The model under review builds one solid part; all positions refer to its coordinate system, in mm. A direction names the side the tool comes from. Round coordinates to 2 decimals unless told otherwise and drop trailing zeros. Write each loop counter-clockwise with the first axis right and the second up, starting at its lowest first coordinate (ties: lowest second). Pieces come first, ordered by that corner, then holes.
Item 1: Add section A-A (y = 9.5). Give the boundary of the cut face in (x, z).
Item 2: Machinability: for faces 5 (the face through (-96, -3.863, 2)), 6 (the face through (-38, 34, 0)), 7 (the face through (-36, -30.276, 2)), which of the approach directions +Z, -Z, +X, -X, +Y, -Y give a long, thin tool a straight path to every point of the face, cutting with its end or side? Answer none if there is none.
Item 3: To check wall thickness, follow L1, parallel to Y at x = -64, z = 3.15; L2, parallel to X at y = 54, z = 1.35; L3, parallel to X at y = 34.5, z = 3.25. State the ranges of each line that lie inside material, in increasing order.
Item 4: Add section D-D (x = -30). Give the boundary of the cut face in (y, z).
Item 5: Add section B-B (x = -85). Give the boundary of the cut face in (y, z), plus the area to 3 significant figures.
Item 6: Add section C-C (z = 2.4). Give the boundary of the cut face in (x, y), plus the area to 4 significant figures.
Item 7: Draft analysis for pull direction X (two halves, no side actions). For faces 1 (the face through (100, -1, 2)), 2 (the face through (-38, 34, 4)), 3 (the face through (-63, -33.276, 2)), 4 (the face through (-100, -40, 2)), state which applies: +X half, -X half, draft (parallel to the pull), parting line (faces both ways), or undercut.
```python
from build123d import *

# Parameters (mm, degrees)
F0_W     = 200
F0_H     = 150
F1_DEPTH = 4
F2_W     = 10
F2_H     = 12.5
F3_DEPTH = 25


with BuildPart() as f1:
    # F0 (on Top) → F1 (new body)
    with BuildSketch(Plane.XY):
        Rectangle(F0_W, F0_H)
    extrude(amount=F1_DEPTH)

    # F2 (on face) → F3 (cut)
    with BuildSketch(Plane.XY.offset(4)):
        Polygon((87.4994372893, -64.5627596692), (87.4994372893, 60.4372403308), (-87.5005627107, 60.4372403308), (-87.5005627107, 34.7239444211), (-41.0005627107, 34.7239444211), (-33.5005627107, 34.7239444211), (-33.5005627107, 26.7239444211), (-38.5005627107, 26.7239444211), (-38.5005627107, 29.7239444211), (-46.0005627107, 29.7239444211), (-87.5005627107, 29.7239444211), (-87.5005627107, 2.7372403308), (-92.5005627107, -0.2627596692), (-100, -0.2627596692), (-100, -3.8627596692), (-92.5005627107, -3.8627596692), (-87.5005627107, -6.8627596692), (-87.5005627107, -33.2760555789), (-38.5005627107, -33.2760555789), (-38.5005627107, -30.2760555789), (-33.5005627107, -30.2760555789), (-33.5005627107, -38.2760555789), (-41.0005627107, -38.2760555789), (-46.0005627107, -38.2760555789), (-87.5005627107, -38.2760555789), (-87.5005627107, -64.5627596692), (-77.5005627107, -64.5627596692), align=None)
        with BuildLine():
            Line((-77.3623862099, 50.4372403308), (-74.3623862099, 50.4372403308))
            Line((-74.3623862099, 50.4372403308), (60.6376137901, 50.4372403308))
            Line((60.6376137901, 50.4372403308), (74.4994372893, 50.4372403308))
            Line((74.4994372893, 50.4372403308), (77.4994372893, 50.4372403308))
            Line((77.4994372893, 50.4372403308), (77.4994372893, 47.4372403308))
            Line((77.4994372893, 47.4372403308), (77.4994372893, -54.5627596692))
            Line((77.4994372893, -54.5627596692), (60.6376137901, -54.5627596692))
            Line((60.6376137901, -54.5627596692), (-77.5005627107, -54.5627596692))
            Line((-77.5005627107, -54.5627596692), (-77.5005627107, -51.5627596692))
            Line((-77.5005627107, -51.5627596692), (60.6376137901, -51.5627596692))
            Line((60.6376137901, -51.5627596692), (69.4994372893, -51.5627596692))
            ThreePointArc((69.4994372893, -51.5627596692), (73.0349711952, -50.0982935751), (74.4994372893, -46.5627596692))
            Line((74.4994372893, -46.5627596692), (74.4994372893, 42.4372403308))
            ThreePointArc((74.4994372893, 42.4372403308), (73.0349711952, 45.9727742368), (69.4994372893, 47.4372403308))
            Line((69.4994372893, 47.4372403308), (60.6376137901, 47.4372403308))
            Line((60.6376137901, 47.4372403308), (57.6376137901, 47.4372403308))
            Line((57.6376137901, 47.4372403308), (-74.3623862099, 47.4372403308))
            Line((-74.3623862099, 47.4372403308), (-77.3623862099, 47.4372403308))
            Line((-77.3623862099, 47.4372403308), (-77.3623862099, 50.4372403308))
        make_face(mode=Mode.SUBTRACT)
        Polygon((39.9994372893, -27.0627596692), (39.9994372893, -2.0627596692), (39.9994372893, 22.9372403308), (39.9994372893, 35.4372403308), (49.9994372893, 35.4372403308), (49.9994372893, 22.9372403308), (49.9994372893, -27.0627596692), (49.9994372893, -39.5627596692), (39.9994372893, -39.5627596692), align=None, mode=Mode.SUBTRACT)
        with BuildLine():
            Line((60.6376137901, 50.4372403308), (-74.3623862099, 50.4372403308))
            Line((-74.3623862099, 50.4372403308), (-77.3623862099, 50.4372403308))
            Line((-77.3623862099, 50.4372403308), (-77.3623862099, 47.4372403308))
            Line((-77.3623862099, 47.4372403308), (-74.3623862099, 47.4372403308))
            Line((-74.3623862099, 47.4372403308), (57.6376137901, 47.4372403308))
            Line((57.6376137901, 47.4372403308), (60.6376137901, 47.4372403308))
            Line((60.6376137901, 47.4372403308), (69.4994372893, 47.4372403308))
            ThreePointArc((69.4994372893, 47.4372403308), (73.0349711952, 45.9727742368), (74.4994372893, 42.4372403308))
            Line((74.4994372893, 42.4372403308), (74.4994372893, -46.5627596692))
            ThreePointArc((74.4994372893, -46.5627596692), (73.0349711952, -50.0982935751), (69.4994372893, -51.5627596692))
            Line((69.4994372893, -51.5627596692), (60.6376137901, -51.5627596692))
            Line((60.6376137901, -51.5627596692), (-77.5005627107, -51.5627596692))
            Line((-77.5005627107, -51.5627596692), (-77.5005627107, -54.5627596692))
            Line((-77.5005627107, -54.5627596692), (60.6376137901, -54.5627596692))
            Line((60.6376137901, -54.5627596692), (77.4994372893, -54.5627596692))
            Line((77.4994372893, -54.5627596692), (77.4994372893, 47.4372403308))
            Line((77.4994372893, 47.4372403308), (77.4994372893, 50.4372403308))
            Line((77.4994372893, 50.4372403308), (74.4994372893, 50.4372403308))
            Line((74.4994372893, 50.4372403308), (60.6376137901, 50.4372403308))
        make_face()
        with Locations((44.9994372893, 29.1872403308)):
            Rectangle(F2_W, F2_H)
        Polygon((39.9994372893, 22.9372403308), (39.9994372893, -2.0627596692), (39.9994372893, -27.0627596692), (49.9994372893, -27.0627596692), (49.9994372893, 22.9372403308), align=None)
        with Locations((44.9994372893, -33.3127596692)):
            Rectangle(F2_W, F2_H)
    extrude(amount=-F3_DEPTH, mode=Mode.SUBTRACT)


solid = f1.part
```
Numbers:
1. outline: (-100, 0) - (-87.5, 0) - (-87.5, 4) - (-100, 4) - close; (87.5, 0) - (100, 0) - (100, 4) - (87.5, 4) - close
2. face 5: +Z, -Z, -X
2. face 6: -Z, +X, -X, +Y, -Y
2. face 7: +Z, -Z
3. L1: y = -75 to -64.56, -38.28 to -33.28, 29.72 to 34.72, 60.44 to 75
3. L2: x = -100 to -87.5, 87.5 to 100
3. L3: x = -100 to -33.5, 87.5 to 100
4. outline: (-75, 0) - (-64.56, 0) - (-64.56, 4) - (-75, 4) - close; (60.44, 0) - (75, 0) - (75, 4) - (60.44, 4) - close
5. outline: (-75, 0) - (-64.56, 0) - (-64.56, 4) - (-75, 4) - close; (-38.28, 0) - (-33.28, 0) - (-33.28, 4) - (-38.28, 4) - close; (29.72, 0) - (34.72, 0) - (34.72, 4) - (29.72, 4) - close; (60.44, 0) - (75, 0) - (75, 4) - (60.44, 4) - close
5. area: 140 mm2
6. outline: (-100, -75) - (100, -75) - (100, 75) - (-100, 75) - (-100, -0.26) - (-92.5, -0.26) - (-87.5, 2.74) - (-87.5, 29.72) - (-38.5, 29.72) - (-38.5, 26.72) - (-33.5, 26.72) - (-33.5, 34.72) - (-87.5, 34.72) - (-87.5, 60.44) - (87.5, 60.44) - (87.5, -64.56) - (-87.5, -64.56) - (-87.5, -38.28) - (-33.5, -38.28) - (-33.5, -30.28) - (-38.5, -30.28) - (-38.5, -33.28) - (-87.5, -33.28) - (-87.5, -6.86) - (-92.5, -3.86) - (-100, -3.86) - close
6. area: 8,635 mm2
7. face 1: +X half
7. face 2: draft
7. face 3: undercut
7. face 4: -X half
